Autodesk Inventor part; units mm, degrees
ref_plane "YZ Plane" through (0, 0, 0) normal (1, 0, 0) x (0, 1, 0)
ref_plane "XZ Plane" through (0, 0, 0) normal (0, 1, 0) x (-1, 0, 0)
ref_plane "XY Plane" through (0, 0, 0) normal (0, 0, 1) x (1, 0, 0)
sketch "Esquisse1" plane through (0, 0, 0) normal (0, 0, 1) x (1, 0, 0)
  line L0 (0, 0) -> (0, 2.5152)
  line L1 (2, -2.5) -> (2, 2.5)
  line L2 (2, 2.5) -> (8, 2.5)
  line L3 (8, 2.5) -> (7.4224, 0.5747)
  line L4 (7.4224, -0.5747) -> (8, -2.5)
  line L5 (8, -2.5) -> (2, -2.5)
  arc A0 (7.4224, 0.5747) -> (7.4224, -0.5747) centre (9.3381, 0) ccw
  point P0 (7.25, 0)
  dimension "d0" = 4
  dimension "d1" = 5
  dimension "d2" = 2.5
  dimension "d3" = 16
  dimension "d4" = 14.5
  dimension "d5" = 2
revolve "Révolution1" add sketch "Esquisse1" angle 360 about axis through (0, 0, 0) along (0, 1, 0)
chamfer "Chanfrein1" distance 0.5 angle 45 2 edges at (-8, 2.5, 0) (-8, -2.5, 0)
equation "\"d2\" = 0.5 * d1"
properties part number "Roulement a bille 634ZZ" material "----------"
Source: CAD feature listing. Evaluate the final solid. Frame: model axes, mm. Round coordinates to 2 decimals unless told otherwise and drop trailing zeros. Loops run counter-clockwise (first coordinate to the right, second up) from the corner with the lowest first, then second, coordinate; pieces in that order, holes last. Notation, with made-up numbers: (-6.5, -30.75) -> (36.5, -30.75) arc R14 ccw to (36.5, -24.75) -> close; hole circle Ø10 at (21.25, 34). An arc over 180 degrees is marked (long way). Answer as a JSON object with one key per item and string values. Group by question number.
Q1. Section query C-C (y = 1.4). Output: boundary loops of the cut face in (x, z).
Q2. Mould query, pull axis X, two halves, no side actions, for faces 1 (the flat face through (2, 2.5, 2)), 2 (the cylindrical face through (0, 0, 2)). Classes: pulls with the +X half, pulls with the -X half, needs draft (parallel to the pull), parting line crosses it, or undercut.
Q3. Ray query, line 1 (Z direction, x = 0, y = 0.8); line 2 (X direction, y = 0.35, z = 0.25); line 3 (Z direction, x = 0, y = -0.4). Return the intervals inside material, ascending. Write a range as from..to.
Q4. Contact query for flat-ended pins moving along their axis: P1, Ø3.5, axis at x = 0, z = 0, coming from the -Y side; P2, Ø1.5, axis at x = -6, z = -6, coming from the -Y side. Output: stop coordinate, or through.
Q5. Section query A-A (z = 0). Output: boundary loops of the cut face in (x, y), plus the area to 3 significant figures.
Q6. Section query B-B (x = 0). Output: boundary loops of the cut face in (y, z), plus the area to 3 significant figures.
Completed:
{
 "1": {"outline": "circle Ø15.34 at (0, 0); hole circle Ø4 at (0, 0)"},
 "2": {"face 1": "needs draft", "face 2": "undercut"},
 "3": {"line 1": "-7.49..-2, 2..7.49", "line 2": "-7.36..-1.98, 1.98..7.36", "line 3": "-7.38..-2, 2..7.38"},
 "4": {"P1": "through", "P2": "y = -2.18"},
 "5": {"outline": "(-7.86, -2.02) -> (-7.5, -2.5) -> (-2, -2.5) -> (-2, 2.5) -> (-7.5, 2.5) -> (-7.86, 2.02) -> (-7.42, 0.57) arc R2 cw to (-7.42, -0.57) -> close; (2, -2.5) -> (7.5, -2.5) -> (7.86, -2.02) -> (7.42, -0.57) arc R2 cw to (7.42, 0.57) -> (7.86, 2.02) -> (7.5, 2.5) -> (2, 2.5) -> close", "area": "55.8 mm²"},
 "6": {"outline": "(-2.5, -7.5) -> (-2.02, -7.86) -> (-0.57, -7.42) arc R2 cw to (0.57, -7.42) -> (2.02, -7.86) -> (2.5, -7.5) -> (2.5, -2) -> (-2.5, -2) -> close; (-2.5, 2) -> (2.5, 2) -> (2.5, 7.5) -> (2.02, 7.86) -> (0.57, 7.42) arc R2 cw to (-0.57, 7.42) -> (-2.02, 7.86) -> (-2.5, 7.5) -> close", "area": "55.8 mm²"}
}
